from build123d import *

# Parameters (mm, degrees)
SKETCH_1_R          = 3
EXTRUDE_1_DEPTH     = 8
SKETCH_2_W          = 18
SKETCH_2_H          = 4
CUT_EXTRUDE_1_DEPTH = 36.09985755


with BuildPart() as part:
    # 草图1 → 凸台-拉伸1 (new body)
    with BuildSketch(Plane.XY):
        with BuildLine():
            Line((-26, 6), (26, 6))
            ThreePointArc((26, 6), (32, 0), (26, -6))
            Line((26, -6), (-26, -6))
            ThreePointArc((-26, -6), (-32, 0), (-26, 6))
        make_face()
        with Locations((-26, 0)):
            Circle(SKETCH_1_R, mode=Mode.SUBTRACT)
        with Locations((26, 0)):
            Circle(SKETCH_1_R, mode=Mode.SUBTRACT)
    extrude(amount=EXTRUDE_1_DEPTH)

    # 草图2 → 切除-拉伸1 (cut, through all)
    with BuildSketch(Plane(origin=(0, 6, 0), x_dir=(1, 0, 0), z_dir=(0, 1, 0))):
        with Locations((-23, -4)):
            Rectangle(SKETCH_2_W, SKETCH_2_H)
    extrude(amount=-CUT_EXTRUDE_1_DEPTH, mode=Mode.SUBTRACT)


solid = part.part
CAD build for the part. Positions are in the model's coordinates, mm. A direction names the side the tool comes from. Round coordinates to 2 decimals unless told otherwise and drop trailing zeros. Write each loop counter-clockwise with the first axis right and the second up, starting at its lowest first coordinate (ties: lowest second). Pieces come first, ordered by that corner, then holes.
(1) Slice it at A-A, the plane y = 0. Write the cut outline in (x, z), and give its area (3 significant figures).
(2) Slice it at C-C, the plane x = 27.5. Write the cut outline in (y, z).
(3) Drop flat-ended pins along their axis: P1, Ø3.5, axis at x = -26, y = 0, coming from the +Z side; P2, Ø3.5, axis at x = -26, y = 1.5, coming from the -Z side. Give the stop position or say it passes through.
(4) Mould opens along Y. For faces 3 (the face through (-29, 0, 1)), 4 (the face through (-21, 0, 6)), 5 (the face through (-32, 0, 1)) say: pulls with the +Y half, pulls with the -Y half, needs draft (parallel to the pull), parting line crosses it, or undercut.
(5) Probe line 1 along Y through (x, z) = (-26, 7.6); line 2 along Z through (x, y) = (-17, 0); line 3 along X through (y, z) = (2, 4.75). List the from-to ranges inside material, lowest first.
(6) Slice it at B-B, the plane z = 7.25. Write the cut outline in (x, y).
(7) 3-axis set-ups, long thin cutter, end or side, ignore diameter. For faces 1 (the face through (-14, 0, 4)), 2 (the face through (0, 0, 8)): which of +Z, -Z, +X, -X, +Y, -Y reach the whole face in a straight line?
From the geometry:
1. outline: (-32, 0) - (-29, 0) - (-29, 2) - (-32, 2) - close; (-32, 6) - (-29, 6) - (-29, 8) - (-32, 8) - close; (-23, 0) - (23, 0) - (23, 8) - (-23, 8) - (-23, 6) - (-14, 6) - (-14, 2) - (-23, 2) - close; (29, 0) - (32, 0) - (32, 8) - (29, 8) - close
1. area: 368 mm2
2. outline: (-5.81, 0) - (-2.6, 0) - (-2.6, 8) - (-5.81, 8) - close; (2.6, 0) - (5.81, 0) - (5.81, 8) - (2.6, 8) - close
3. P1: passes through
3. P2: stops at z = 0
4. face 3: undercut
4. face 4: needs draft
4. face 5: parting line crosses it
5. line 1: y = -6 to -3, 3 to 6
5. line 2: z = 0 to 2, 6 to 8
5. line 3: x = -14 to 23.76, 28.24 to 31.66
6. outline: (-26, -6) - (26, -6) arc R6 ccw to (26, 6) - (-26, 6) arc R6 ccw to start; hole circle Ø6 at (-26, 0); hole circle Ø6 at (26, 0)
7. face 1: -X, +Y, -Y
7. face 2: +Z, +X, -X, +Y, -Y
